Input: part model. Units: mm. Frame: model coordinates. A direction names the side the tool comes from. Give positions to 0.01 mm unless a question says otherwise; leave off trailing zeros. Write each loop counter-clockwise with the first axis right and the second up, starting at its lowest first coordinate (ties: lowest second). Pieces come first, ordered by that corner, then holes. Notation, with made-up numbers: (37.25, 88) - (41.25, 88) arc R8 cw to (41.25, 94) - close; hole circle Ø4 at (14.5, -10.75). An arc over 180 degrees is marked (long way). Use a Markdown table: item, result. Add a question column.
1. Section query D-D, the plane x = -10. Return loops of the section in (y, z), plus the area to 3 significant figures.
2. Section query B-B, the plane z = 2.05. Return loops of the section in (x, y).
3. Pin query (flat end, axial travel): pin 1 (1.5 mm diameter, centred on x = 0.5, z = 4.5, fed in from -Y). Return the tip coordinate at first contact, or that it passes through.
4. Section query C-C, the plane y = 10. Return loops of the section in (x, z), plus the area to 3 significant figures.
5. Mould query, pull axis X, two halves, no side actions, for faces 1 (the cylindrical face through (-4.336, -19.524, 2.465)), 2 (the cylindrical face through (0, -13, 2)), 3 (the flat face through (0, 0, 5)), 4 (the cylindrical face through (-10.2, 4.7, 2.5)). Classes: released by +X, released by -X, zero draft, split by the parting line, or undercut.
6. Set-up query: faces 5 (the cylindrical face through (0, -9, 2)), 6 (the flat face through (0, 0, 0)). Return all of +Z, -Z, +X, -X, +Y, -Y with unobstructed straight access to the full face (end or side cutting, diameter ignored); none if empty.
7. Material intervals for probe 1 along X at (y, z) = (-6, 2.35); probe 2 along X at (y, z) = (-7.5, 4.3); probe 3 along Y at (x, z) = (2, 3.45), sorted ascending.
8. Section query A-A, the plane x = 0. Return loops of the section in (y, z).
```python
from build123d import *

# Parameters (mm, degrees)
SKETCH_R      = 20
EXTRUDE_DEPTH = 5


with BuildPart() as part:
    # Sketch → Extrude (new body)
    with BuildSketch(Plane.XY):
        Circle(SKETCH_R)
        with BuildLine():
            ThreePointArc((7.372368, 5.162188), (0, 9), (-7.372368, 5.162188))
            ThreePointArc((-10.648977, 7.456494), (-10.157825, 4.671037), (-7.372368, 5.162188))
            ThreePointArc((10.648977, 7.456494), (0, 13), (-10.648977, 7.456494))
            ThreePointArc((7.372368, 5.162188), (10.157825, 4.671037), (10.648977, 7.456494))
        make_face(mode=Mode.SUBTRACT)
        with BuildLine():
            ThreePointArc((-7.372368, -5.162188), (0, -9), (7.372368, -5.162188))
            ThreePointArc((10.648977, -7.456494), (10.157825, -4.671037), (7.372368, -5.162188))
            ThreePointArc((-10.648977, -7.456494), (0, -13), (10.648977, -7.456494))
            ThreePointArc((-7.372368, -5.162188), (-10.157825, -4.671037), (-10.648977, -7.456494))
        make_face(mode=Mode.SUBTRACT)
    extrude(amount=EXTRUDE_DEPTH)


solid = part.part
```
Result sheet:
| question | item | result |
|---|---|---|
| 1 | outline | (-17.32, 0) - (-8.31, 0) - (-8.31, 5) - (-17.32, 5) - close; (-4.57, 0) - (4.57, 0) - (4.57, 5) - (-4.57, 5) - close; (8.31, 0) - (17.32, 0) - (17.32, 5) - (8.31, 5) - close |
| 1 | area | 136 mm² |
| 2 | outline | circle Ø40 at (0, 0); hole (-10.65, -7.46) arc R13 ccw to (10.65, -7.46) arc R2 ccw to (7.37, -5.16) arc R9 cw to (-7.37, -5.16) arc R2 ccw to start; hole (-10.65, 7.46) arc R2 ccw to (-7.37, 5.16) arc R9 cw to (7.37, 5.16) arc R2 ccw to (10.65, 7.46) arc R13 ccw to start |
| 3 | pin 1 | stops at y = -20 |
| 4 | outline | (-17.32, 0) - (-8.31, 0) - (-8.31, 5) - (-17.32, 5) - close; (8.31, 0) - (17.32, 0) - (17.32, 5) - (8.31, 5) - close |
| 4 | area | 90.1 mm² |
| 5 | face 1 | split by the parting line |
| 5 | face 2 | undercut |
| 5 | face 3 | zero draft |
| 5 | face 4 | undercut |
| 6 | face 5 | +Z, -Z |
| 6 | face 6 | -Z, +X, -X, +Y, -Y |
| 7 | probe 1 | x = -19.08 to -10.99, -6.71 to 6.71, 10.99 to 19.08 |
| 7 | probe 2 | x = -18.54 to -10.62, -4.97 to 4.97, 10.62 to 18.54 |
| 7 | probe 3 | y = -19.9 to -12.85, -8.77 to 8.77, 12.85 to 19.9 |
| 8 | outline | (-20, 0) - (-13, 0) - (-13, 5) - (-20, 5) - close; (-9, 0) - (9, 0) - (9, 5) - (-9, 5) - close; (13, 0) - (20, 0) - (20, 5) - (13, 5) - close |
